Source: CAD feature listing. Evaluate the final solid. Frame: model axes, mm. A direction names the side the tool comes from. Give positions to 0.01 mm unless a question says otherwise; leave off trailing zeros. Use one line per item in the form item = value. Start each with the question number.
(1) Material intervals for line 1 along X through (y, z) = (9.5, -13); line 2 along X through (y, z) = (6.5, 8.5); line 3 along X through (y, z) = (7.5, 1), sorted ascending. Write a range as from..to.
(2) Cut plane A-A, the plane y = 8.75. Count the separate pieces of the cut face and the enclosed holes in it, and give its area (3 significant figures).
(3) First-contact query: P1, Ø3, axis at x = 23, z = -28.5, coming from the +Y side; P2, Ø4, axis at y = 1.5, z = -7, coming from the -X side; P3, Ø8, axis at x = -1, z = 9, coming from the +Y side; P4, Ø5, axis at x = 23, z = 28.5, coming from the +Y side. Flat tips, straight axial feed; report the tip coordinate or a pass-through.
(4) Set-up query: faces 1 (the face through (-18.39, 5.48, -39.9)), 2 (the face through (19.997, 8.156, -29.745)). Return all of +Z, -Z, +X, -X, +Y, -Y with unobstructed straight access to the full face (end or side cutting, diameter ignored); none if empty.
from build123d import *

# Parameters (mm, degrees)
SKETCH1_R                                       = 50.8
SKETCH1_R_2                                     = 19.25
BOSS_EXTRUDE1_DEPTH                             = 6.35
SKETCH2_R                                       = 50.8
SKETCH2_R_2                                     = 30
BOSS_EXTRUDE2_DEPTH                             = 4.7625
SKETCH3_R                                       = 3
CUT_EXTRUDE1_DEPTH                              = 4.7625
CHAMFER1_SIZE                                   = 1.2
M4X0_7_TAPPED_HOLE1_D                           = 3.3
M4X0_7_TAPPED_HOLE1_DEPTH                       = 11.1135
BOSS_EXTRUDE3_START                             = -6.35
SKETCH13_R                                      = 19.25
SKETCH13_R_2                                    = 14.25
BOSS_EXTRUDE3_DEPTH                             = 6.35
CSK_FOR_M3_FLAT_HEAD_MACHINE_SCREW1_D           = 3.4
CSK_FOR_M3_FLAT_HEAD_MACHINE_SCREW1_CSINK_D     = 6.3
CSK_FOR_M3_FLAT_HEAD_MACHINE_SCREW1_CSINK_ANGLE = 90
CUT_EXTRUDE4_DEPTH                              = 73.696407451
CUT_EXTRUDE4_DEPTH_BACK                         = 73.696407451


with BuildPart() as part:
    # Sketch1 → Boss-Extrude1 (new body)
    with BuildSketch(Plane(origin=(0, 0, 0), x_dir=(1, 0, 0), z_dir=(0, 1, 0))):
        with Locations(Location((0, 0, 0), (0, 0, 270))):
            Circle(SKETCH1_R)
        with Locations(Location((0, 0, 0), (0, 0, 270))):
            Circle(SKETCH1_R_2, mode=Mode.SUBTRACT)
    extrude(amount=BOSS_EXTRUDE1_DEPTH)

    # Sketch2 → Boss-Extrude2 (add)
    with BuildSketch(Plane(origin=(0, 6.35, 0), x_dir=(1, 0, 0), z_dir=(0, 1, 0))):
        with Locations(Location((0, 0, 0), (0, 0, 270))):
            Circle(SKETCH2_R)
        with Locations(Location((0, 0, 0), (0, 0, 90))):
            Circle(SKETCH2_R_2, mode=Mode.SUBTRACT)
    extrude(amount=BOSS_EXTRUDE2_DEPTH)

    # Sketch3 → Cut-Extrude1 (cut)
    with BuildSketch(Plane(origin=(0, 11.1125, 0), x_dir=(1, 0, 0), z_dir=(0, 1, 0))):
        with Locations(Location((35, 0, 0), (0, 0, 270))):
            Circle(SKETCH3_R)
        with Locations(Location((33.445048203, -10.316431104, 0), (0, 0, 270))):
            Circle(SKETCH3_R)
        with Locations(Location((28.918357101, -19.716202032, 0), (0, 0, 270))):
            Circle(SKETCH3_R)
        with Locations(Location((21.822143065, -27.364101886, 0), (0, 0, 270))):
            Circle(SKETCH3_R)
        with Locations(Location((12.786935853, -32.580581203, 0), (0, 0, 270))):
            Circle(SKETCH3_R)
        with Locations(Location((2.615553276, -34.902132901, 0), (0, 0, 270))):
            Circle(SKETCH3_R)
        with Locations(Location((-7.788232688, -34.122476926, 0), (0, 0, 270))):
            Circle(SKETCH3_R)
        with Locations(Location((-17.5, -30.310889132, 0), (0, 0, 270))):
            Circle(SKETCH3_R)
        with Locations(Location((-25.656815514, -23.806045822, 0), (0, 0, 270))):
            Circle(SKETCH3_R)
        with Locations(Location((-31.533910377, -15.185930869, 0), (0, 0, 270))):
            Circle(SKETCH3_R)
        with Locations(Location((-34.609078918, -5.216479316, 0), (0, 0, 270))):
            Circle(SKETCH3_R)
        with Locations(Location((-34.609078918, 5.216479316, 0), (0, 0, 270))):
            Circle(SKETCH3_R)
        with Locations(Location((-31.533910377, 15.185930869, 0), (0, 0, 270))):
            Circle(SKETCH3_R)
        with Locations(Location((-25.656815514, 23.806045822, 0), (0, 0, 270))):
            Circle(SKETCH3_R)
        with Locations(Location((-17.5, 30.310889132, 0), (0, 0, 270))):
            Circle(SKETCH3_R)
        with Locations(Location((-7.788232688, 34.122476926, 0), (0, 0, 270))):
            Circle(SKETCH3_R)
        with Locations(Location((2.615553276, 34.902132901, 0), (0, 0, 270))):
            Circle(SKETCH3_R)
        with Locations(Location((12.786935853, 32.580581203, 0), (0, 0, 270))):
            Circle(SKETCH3_R)
        with Locations(Location((21.822143065, 27.364101886, 0), (0, 0, 270))):
            Circle(SKETCH3_R)
        with Locations(Location((28.918357101, 19.716202032, 0), (0, 0, 270))):
            Circle(SKETCH3_R)
        with Locations(Location((33.445048203, 10.316431104, 0), (0, 0, 270))):
            Circle(SKETCH3_R)
    extrude(amount=-CUT_EXTRUDE1_DEPTH, mode=Mode.SUBTRACT)

    # Chamfer1
    chamfer1_edges = [part.edges().sort_by_distance(p)[0] for p in [
        (2.615553276, 11.1125, 31.902132901),
        (12.786935853, 11.1125, 29.580581203),
        (21.822143065, 11.1125, 24.364101886),
        (28.918357101, 11.1125, 16.716202032),
        (33.445048203, 11.1125, 7.316431104),
        (35, 11.1125, -3),
        (33.445048203, 11.1125, -13.316431104),
        (28.918357101, 11.1125, -22.716202032),
        (21.822143065, 11.1125, -30.364101886),
        (12.786935853, 11.1125, -35.580581203),
        (2.615553276, 11.1125, -37.902132901),
        (-7.788232688, 11.1125, -37.122476926),
        (-17.5, 11.1125, -33.310889132),
        (-25.656815514, 11.1125, -26.806045822),
        (-31.533910377, 11.1125, -18.185930869),
        (-34.609078918, 11.1125, -8.216479316),
        (-7.788232688, 11.1125, 31.122476926),
        (-17.5, 11.1125, 27.310889132),
        (-25.656815514, 11.1125, 20.806045822),
        (-31.533910377, 11.1125, 12.185930869),
        (-34.609078918, 11.1125, 2.216479316),
    ]]
    chamfer(chamfer1_edges, length=CHAMFER1_SIZE)

    # M4x0.7 Tapped Hole1
    with Locations(Plane(origin=(0, 11.1125, 0), x_dir=(1, 0, 0), z_dir=(0, 1, 0))):
        with Locations((0, -45.4), (0, 0), (-19.698321756, 40.903986603), (19.698321756, 40.903986603), (44.261727213, 10.102450402), (35.495149304, -28.306437004), (-35.495149304, -28.306437004), (-44.261727213, 10.102450402)):
            Hole(M4X0_7_TAPPED_HOLE1_D / 2, depth=M4X0_7_TAPPED_HOLE1_DEPTH)

    # Sketch13 → Boss-Extrude3 (add)
    with BuildSketch(Plane(origin=(0, 6.35, 0), x_dir=(1, 0, 0), z_dir=(0, 1, 0)).offset(BOSS_EXTRUDE3_START)):
        Circle(SKETCH13_R)
        with Locations(Location((0, 0, 0), (0, 0, 270))):
            Circle(SKETCH13_R_2, mode=Mode.SUBTRACT)
    extrude(amount=BOSS_EXTRUDE3_DEPTH)

    # CSK for M3 Flat Head Machine Screw1 (through all)
    with Locations(Plane(origin=(0, 6.35, 0), x_dir=(1, 0, 0), z_dir=(0, 1, 0))):
        with Locations((8.677674782, 18.019377358), (-18.019377358, 8.677674782), (18.019377358, -8.677674782), (-8.677674782, -18.019377358)):
            CounterSinkHole(CSK_FOR_M3_FLAT_HEAD_MACHINE_SCREW1_D / 2, CSK_FOR_M3_FLAT_HEAD_MACHINE_SCREW1_CSINK_D / 2, counter_sink_angle=CSK_FOR_M3_FLAT_HEAD_MACHINE_SCREW1_CSINK_ANGLE)

    # Sketch16 → Cut-Extrude4 (cut, two sides: drawn at the far end of the back side and taken through both)
    with BuildSketch(Plane(origin=(0, 11.1125, 0), x_dir=(1, 0, 0), z_dir=(0, 1, 0)).offset(-CUT_EXTRUDE4_DEPTH_BACK)):
        Polygon((-20.93922925, -43.480757565), (12.568971471, -59.617456554), (3.715578601, -78.001716282), (-56.57071251, -48.969368621), (-47.717319639, -30.585108893), align=None)
    extrude(amount=CUT_EXTRUDE4_DEPTH + CUT_EXTRUDE4_DEPTH_BACK, mode=Mode.SUBTRACT)


solid = part.part
Geometry says:
q1.line_1 = -49.11..-33.59, -29.48..-27.04, 27.04..32.1, 34.79..49.11
q1.line_2 = -50.08..-28.77, 28.77..31.06, 35.83..50.08
q1.line_3 = -50.79..-29.98, 29.98..32.17, 37.83..50.79
q2.separate_pieces = 1
q2.enclosed_holes = 29
q2.area = 4,570 mm^2
q3.P1 = 10.05
q3.P2 = -50.55
q3.P3 = through
q3.P4 = 11.05
q4.face_1 = +Y, -Y
q4.face_2 = +Y
